Design review of the part built by this model. Coordinates are the model's own, in mm. Face numbers are marked on the shaded views. A direction names the side the tool comes from. Coordinates: 2 decimals unless noted, no trailing zeros. Loops run counter-clockwise (first coordinate to the right, second up) from the corner with the lowest first, then second, coordinate; pieces in that order, holes last. Notation, with made-up numbers: (38.25, 4.5) -> (69.25, 4.5) arc R18 cw to (69.25, 20.5) -> close; hole circle Ø2 at (-11.75, 59.25). An arc over 180 degrees is marked (long way). Use a Markdown table: item, result. Add a question column.
Q1. Clearance check with flat-ended pins moving along their axes: pin 1 Ø4 at (x, z) = (21.5, 1.5) entering from -Y; pin 2 Ø1.5 at (x, y) = (-2, 3.5) entering from +Z; pin 3 Ø3 at (x, z) = (38.5, 8) entering from +Y. State where each tip first meets the part, or that it passes through.
Q2. Take a section at A-A on z = 3. Write out the cut boundary in (x, y), plus the area to 3 significant figures.
Q3. For probe 1 along X at (y, z) = (-1.5, 5); probe 2 along X at (y, z) = (1.25, 10); probe 3 along Y at (x, z) = (-37, 3), list the stretches that pass through material, from the lowest coordinate up.
Q4. For the marked faces 5 and 6, list the 3-axis set-ups (+Z, -Z, +X, -X, +Y, -Y) from which the entire face can be reached by the end or side of a thin tool; tool diameter is ignored.
Q5. Take a section at B-B on y = -1.5. Write out the cut boundary in (x, z).
Q6. Take a section at D-D on x = 37. Write out the cut boundary in (y, z), plus the area to 3 significant figures.
Q7. Take a section at C-C on z = 9.5. Write out the cut boundary in (x, y), plus the area to 3 significant figures.
Q8. Draft analysis for pull direction X (two halves, no side actions). For the marked faces 1, 2, 3 and 4, state which applies: pulls with the +X half, pulls with the -X half, needs draft (parallel to the pull), parting line crosses it, or undercut.
from build123d import *

# Parameters (mm, degrees)
F1_DEPTH = 15
F2_W     = 68
F2_H     = 3
F3_DEPTH = 10
F4_R     = 1.35
F5_DEPTH = 8
F6_W     = 3
F6_H     = 10
F6_R     = 1.35
F7_DEPTH = 80.001


with BuildPart() as f1:
    # F0 (on Top) → F1 (new body)
    with BuildSketch(Plane.XY):
        Polygon((-40, -4.5), (-34, -4.5), (-34, 1.5), (0, 1.5), (34, 1.5), (34, -4.5), (40, -4.5), (40, 4.5), (34, 4.5), (0, 4.5), (-34, 4.5), (-40, 4.5), align=None)
    extrude(amount=F1_DEPTH)

    # F2 (on face) → F3 (cut)
    with BuildSketch(Plane.XY.offset(15)):
        with Locations((0, 3)):
            Rectangle(F2_W, F2_H)
    extrude(amount=-F3_DEPTH, mode=Mode.SUBTRACT)

    # F4 (on face) → F5 (cut)
    with BuildSketch(Plane(origin=(0, 0, 0), x_dir=(1, 0, 0), z_dir=(0, 0, -1))):
        with Locations((37, 1.5)):
            Circle(F4_R)
        with Locations((-37, 1.5)):
            Circle(F4_R)
    extrude(amount=-F5_DEPTH, mode=Mode.SUBTRACT)

    # F6 (on face) → F7 (cut, through all)
    with BuildSketch(Plane.YZ.offset(40)):
        with Locations((3, 10)):
            Rectangle(F6_W, F6_H)
        with Locations((-1.5, 12)):
            Circle(F6_R)
    extrude(amount=-F7_DEPTH, mode=Mode.SUBTRACT)


solid = f1.part
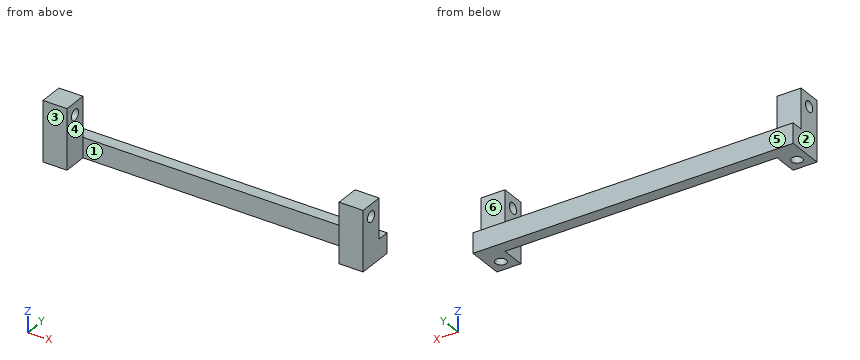
Answer list:
| question | item | result |
|---|---|---|
| 1 | pin 1 | y = 1.5 |
| 1 | pin 2 | z = 5 |
| 1 | pin 3 | y = 1.5 |
| 2 | outline | (-40, -4.5) -> (-34, -4.5) -> (-34, 1.5) -> (34, 1.5) -> (34, -4.5) -> (40, -4.5) -> (40, 4.5) -> (-40, 4.5) -> close; hole circle Ø2.7 at (-37, -1.5); hole circle Ø2.7 at (37, -1.5) |
| 2 | area | 301 mm² |
| 3 | probe 1 | -40 to -38.35, -35.65 to -34, 34 to 35.65, 38.35 to 40 |
| 3 | probe 2 | -40 to -34, 34 to 40 |
| 3 | probe 3 | -4.5 to -2.85, -0.15 to 4.5 |
| 4 | face 5 | +Z, -Z, +X, -X, +Y |
| 4 | face 6 | +Z, +X, -X, +Y |
| 5 | outline | (-40, 0) -> (-38.35, 0) -> (-38.35, 8) -> (-35.65, 8) -> (-35.65, 0) -> (-34, 0) -> (-34, 10.65) -> (-40, 10.65) -> close; (-40, 13.35) -> (-34, 13.35) -> (-34, 15) -> (-40, 15) -> close; (34, 0) -> (35.65, 0) -> (35.65, 8) -> (38.35, 8) -> (38.35, 0) -> (40, 0) -> (40, 10.65) -> (34, 10.65) -> close; (34, 13.35) -> (40, 13.35) -> (40, 15) -> (34, 15) -> close |
| 6 | outline | (-4.5, 0) -> (-2.85, 0) -> (-2.85, 8) -> (-0.15, 8) -> (-0.15, 0) -> (4.5, 0) -> (4.5, 5) -> (1.5, 5) -> (1.5, 15) -> (-4.5, 15) -> close; hole circle Ø2.7 at (-1.5, 12) |
| 6 | area | 77.7 mm² |
| 7 | outline | (-40, -4.5) -> (-34, -4.5) -> (-34, 1.5) -> (-40, 1.5) -> close; (34, -4.5) -> (40, -4.5) -> (40, 1.5) -> (34, 1.5) -> close |
| 7 | area | 72.0 mm² |
| 8 | face 1 | undercut |
| 8 | face 2 | pulls with the -X half |
| 8 | face 3 | needs draft |
| 8 | face 4 | undercut |
